from build123d import *

# Parameters (mm, degrees)
SKETCH_1_R      = 2.6
SKETCH_1_R_2    = 1.6
EXTRUDE_1_DEPTH = 3


with BuildPart() as part:
    # 草图1 → 凸台-拉伸1 (new body)
    with BuildSketch(Plane.XY):
        with BuildLine():
            Line((-60, 77.5), (-5, 77.5))
            ThreePointArc((-5, 77.5), (-1.464466094, 76.035533906), (0, 72.5))
            Line((0, 72.5), (0, -50))
            ThreePointArc((0, -50), (-1.464466094, -53.535533906), (-5, -55))
            Line((-5, -55), (-60, -55))
            ThreePointArc((-60, -55), (-63.535533906, -53.535533906), (-65, -50))
            Line((-65, -50), (-65, -32.5))
            ThreePointArc((-65, -32.5), (-62.071067812, -25.428932188), (-55, -22.5))
            Line((-55, -22.5), (-50, -22.5))
            ThreePointArc((-50, -22.5), (-42.928932188, -19.571067812), (-40, -12.5))
            Line((-40, -12.5), (-40, 47.5))
            ThreePointArc((-40, 47.5), (-42.928932188, 54.571067812), (-50, 57.5))
            Line((-50, 57.5), (-60, 57.5))
            ThreePointArc((-60, 57.5), (-63.535533906, 58.964466094), (-65, 62.5))
            Line((-65, 62.5), (-65, 72.5))
            ThreePointArc((-65, 72.5), (-63.535533906, 76.035533906), (-60, 77.5))
        make_face()
        with Locations((-10, 10)):
            Circle(SKETCH_1_R, mode=Mode.SUBTRACT)
        with Locations((-55, 67.5)):
            Circle(SKETCH_1_R_2, mode=Mode.SUBTRACT)
        with Locations((-30, 10)):
            Circle(SKETCH_1_R_2, mode=Mode.SUBTRACT)
        with Locations((-30, 67.5)):
            Circle(SKETCH_1_R_2, mode=Mode.SUBTRACT)
        with Locations((-42.5, 67.5)):
            Circle(SKETCH_1_R_2, mode=Mode.SUBTRACT)
        with Locations((-30, 47.5)):
            Circle(SKETCH_1_R_2, mode=Mode.SUBTRACT)
        with Locations((-30, 30)):
            Circle(SKETCH_1_R_2, mode=Mode.SUBTRACT)
        with Locations((-55, -32.5)):
            Circle(SKETCH_1_R_2, mode=Mode.SUBTRACT)
        with Locations((-42.5, -32.5)):
            Circle(SKETCH_1_R_2, mode=Mode.SUBTRACT)
        with Locations((-30, -32.5)):
            Circle(SKETCH_1_R_2, mode=Mode.SUBTRACT)
        with Locations((-10, -32.5)):
            Circle(SKETCH_1_R_2, mode=Mode.SUBTRACT)
        with BuildLine():
            Line((-26, -5), (-10, -5))
            ThreePointArc((-10, -5), (-7.171572875, -6.171572875), (-6, -9))
            Line((-6, -9), (-6, -18.5))
            ThreePointArc((-6, -18.5), (-7.171572875, -21.328427125), (-10, -22.5))
            Line((-10, -22.5), (-26, -22.5))
            ThreePointArc((-26, -22.5), (-28.828427125, -21.328427125), (-30, -18.5))
            Line((-30, -18.5), (-30, -9))
            ThreePointArc((-30, -9), (-28.828427125, -6.171572875), (-26, -5))
        make_face(mode=Mode.SUBTRACT)
        with BuildLine():
            Line((-10, 25), (-16, 25))
            ThreePointArc((-16, 25), (-18.828427125, 26.171572875), (-20, 29))
            Line((-20, 29), (-20, 65.5))
            ThreePointArc((-20, 65.5), (-18.828427125, 68.328427125), (-16, 69.5))
            Line((-16, 69.5), (-10, 69.5))
            ThreePointArc((-10, 69.5), (-7.171572875, 68.328427125), (-6, 65.5))
            Line((-6, 65.5), (-6, 29))
            ThreePointArc((-6, 29), (-7.171572875, 26.171572875), (-10, 25))
        make_face(mode=Mode.SUBTRACT)
    extrude(amount=EXTRUDE_1_DEPTH)


solid = part.part
Design review of the part built by this model. Coordinates are the model's own, in mm. A direction names the side the tool comes from. Give positions to 0.01 mm unless a question says otherwise; leave off trailing zeros. Loops run counter-clockwise (first coordinate to the right, second up) from the corner with the lowest first, then second, coordinate; pieces in that order, holes last. Notation, with made-up numbers: (-33.5, 56.5) - (-12.5, 56.5) arc R16 cw to (-12.5, 79.5) - close; hole circle Ø7 at (-25, -31.75). An arc over 180 degrees is marked (long way). Use CSV: the item, a comma, the result in double quotes. Start each with the question number.
1. Machinability: for faces 1 (the cylindrical face through (-7.141, -21.297, 1.479)), 2 (the cylindrical face through (-42.85, 54.49, 1.48)), 3 (the flat face through (-25, 12, 3)), which of the approach directions +Z, -Z, +X, -X, +Y, -Y give a long, thin tool a straight path to every point of the face, cutting with its end or side? Answer none if there is none.
2. Add section A-A (x = -51.5). State the section outline as (y, z) points, plus the area to 4 significant figures.
3. Wall thickness on L1, parallel to X at y = -10.5, z = 2.05; L2, parallel to Y at x = -52, z = 1; L3, parallel to Y at x = -10.5, z = 0.25: over which ranges is each line inside the solid? List them lowest first.
4. Insertion check: P1, Ø0.9, axis at y = 51, z = 1, coming from the -X side; P2, Ø4, axis at x = -42.5, y = 67.5, coming from the +Z side; P3, Ø3, axis at x = -30, y = 47.5, coming from the -Z side; P4, Ø1.5, axis at y = -15.5, z = 2, coming from the -X side. Each pin has a flat end and moves straight along its axis. Give the tip position at first contact, or say it passes through.
5. Draft analysis for pull direction Y (two halves, no side actions). For faces 4 (the cylindrical face through (-1, -53, 1)), 5 (the flat face through (-65, 67, 1)), 6 (the cylindrical face through (-62.15, -25.51, 1.48)), state which applies: released by +Y, released by -Y, zero draft, split by the parting line, or undercut.
6. Add section B-B (y = 67.5). State the section outline as (x, z) points.
7. Add section D-D (z = 0.9). Count the separate pieces of the cut face and the enclosed holes in it, plus the area to 3 significant figures.
8. Add section C-C (x = -42.5). State the section outline as (y, z) points, plus the area to 3 significant figures.
Results found:
1,face 1,"+Z, -Z"
1,face 2,"+Z, -Z, -X"
1,face 3,"+Z, +X, -X, +Y, -Y"
2,outline,"(-55, 0) - (-22.5, 0) - (-22.5, 3) - (-55, 3) - close; (57.5, 0) - (77.5, 0) - (77.5, 3) - (57.5, 3) - close"
2,area,"157.5 mm²"
3,L1,"x = -40 to -30, -6 to 0"
3,L2,"y = -55 to -22.5, 57.5 to 77.5"
3,L3,"y = -55 to -34.02, -30.98 to -22.5, -5 to 7.45, 12.55 to 25, 69.5 to 77.5"
4,P1,"stops at x = -40.81"
4,P2,"stops at z = 3"
4,P3,"passes through"
4,P4,"stops at x = -40.73"
5,face 4,"released by -Y"
5,face 5,"zero draft"
5,face 6,"undercut"
6,outline,"(-65, 0) - (-56.6, 0) - (-56.6, 3) - (-65, 3) - close; (-53.4, 0) - (-44.1, 0) - (-44.1, 3) - (-53.4, 3) - close; (-40.9, 0) - (-31.6, 0) - (-31.6, 3) - (-40.9, 3) - close; (-28.4, 0) - (-19.46, 0) - (-19.46, 3) - (-28.4, 3) - close; (-6.54, 0) - (0, 0) - (0, 3) - (-6.54, 3) - close"
7,separate pieces,"1"
7,enclosed holes,"13"
7,area,"5,490 mm²"
8,outline,"(-55, 0) - (-34.1, 0) - (-34.1, 3) - (-55, 3) - close; (-30.9, 0) - (-19.11, 0) - (-19.11, 3) - (-30.9, 3) - close; (54.11, 0) - (65.9, 0) - (65.9, 3) - (54.11, 3) - close; (69.1, 0) - (77.5, 0) - (77.5, 3) - (69.1, 3) - close"
8,area,"159 mm²"
